from build123d import *

# Parameters (mm, degrees)
CYLINDER002_R     = 0.3
CYLINDER002_DEPTH = 3
CYLINDER001_R     = 0.3
CYLINDER001_DEPTH = 3
BOX001_W          = 1
BOX001_H          = 1
BOX001_DEPTH      = 4
BOX_W             = 1
BOX_H             = 1
BOX_DEPTH         = 4
TORUS_R           = 2.2
CYLINDER_R        = 5.25
CYLINDER_DEPTH    = 14
FILLET_R          = 0.5


with BuildPart() as pin2:
    # Cylinder002 → Cylinder002 (new body)
    with BuildSketch(Plane(origin=(2.5, 0, -3), x_dir=(1, 0, 0), z_dir=(0, 0, 1))):
        Circle(CYLINDER002_R)
    extrude(amount=CYLINDER002_DEPTH)


with BuildPart() as pin1:
    # Cylinder001 → Cylinder001 (new body)
    with BuildSketch(Plane(origin=(-2.5, 0, -3), x_dir=(1, 0, 0), z_dir=(0, 0, 1))):
        Circle(CYLINDER001_R)
    extrude(amount=CYLINDER001_DEPTH)


with BuildPart() as box001:
    # Box001 → Box001 (new body)
    with BuildSketch(Plane(origin=(5, -0.5, 15), x_dir=(1, 0, 0), z_dir=(0, 0, 1))):
        with Locations((0.5, 0.5)):
            Rectangle(BOX001_W, BOX001_H)
    extrude(amount=BOX001_DEPTH)


with BuildPart() as box:
    # Box → Box (new body)
    with BuildSketch(Plane(origin=(5, -0.5, 7), x_dir=(1, 0, 0), z_dir=(0, 0, 1))):
        with Locations((0.5, 0.5)):
            Rectangle(BOX_W, BOX_H)
    extrude(amount=BOX_DEPTH)


with BuildPart() as ring:
    # Torus → Torus (revolve)
    with BuildSketch(Plane(origin=(0, 0, 3.5), x_dir=(1, 0, 0), z_dir=(0, -1, 0))):
        with Locations((7.15, 0)):
            Circle(TORUS_R)
    revolve(axis=Axis((0, 0, 3.5), (0, 0, 1)))


with BuildPart() as obj1:
    # Cylinder → Cylinder (new body)
    with BuildSketch(Plane.XY):
        Circle(CYLINDER_R)
    extrude(amount=CYLINDER_DEPTH)

    # Fillet
    fillet_edges = [obj1.edges().sort_by_distance(p)[0] for p in [
        (-5.25, 0, 14),
        (-5.25, 0, 0),
    ]]
    fillet(fillet_edges, radius=FILLET_R)

    # Cut: cut Ring
    add(ring.part, mode=Mode.SUBTRACT)

    # Cut001: cut Box
    add(box.part, mode=Mode.SUBTRACT)

    # Cut002: cut Box001
    add(box001.part, mode=Mode.SUBTRACT)

    # Fusion: union Pin1+
    add(pin1.part)

    # Fusion001: union Pin2-
    add(pin2.part)


solid = obj1.part
Read the model definition and answer for the solid it produces. Units are mm, in the model's axes. Give positions to 0.01 mm unless a question says otherwise; leave off trailing zeros. Write each loop counter-clockwise with the first axis right and the second up, starting at its lowest first coordinate (ties: lowest second). Pieces come first, ordered by that corner, then holes. Notation, with made-up numbers: (69, 69) - (114, 69) arc R21 cw to (114, 88) - close; hole circle Ø6 at (87, -3). An arc over 180 degrees is marked (long way). Answer in a Markdown table with one row per item. Add a question column.
Item 1: Section C-C, the plane z = 6.75 is taken. Write down the section's boundary in (x, y), and give its area (3 significant figures).
Item 2: Section A-A, the plane y = 0 is taken. Write down the section's boundary in (x, z), and give its area (3 significant figures).
Item 3: Section B-B, the plane x = 0 is taken. Write down the section's boundary in (y, z), and give its area (3 significant figures).
Item 4: Find the intervals of material crossed by L1, parallel to Z at x = 4, y = -2; L2, parallel to Y at x = 2.5, z = -1.5; L3, parallel to X at y = -0.75, z = 2.75, in increasing order.
Item 5: Flat-ended cylindrical pins translate along their axes: P1, Ø3, axis at y = 0, z = 0, coming from the +X side; P2, Ø2, axis at y = 2.5, z = 9.5, coming from the -X side. Find the tip coordinate at first contact, or state that the pin passes through.
Item 6: Determine the mould class of faces 1 (the face through (5, 0, 9)), 2 (the face through (5, 1.6, 9)), 3 (the face through (0, 0, 0)) for opening direction Y: pulls with the +Y half, pulls with the -Y half, needs draft (parallel to the pull), parting line crosses it, or undercut.
Item 7: Section D-D, the plane z = 3.5 is taken. Write down the section's boundary in (x, y).
Recorded:
| question | item | result |
|---|---|---|
| 1 | outline | circle Ø10.5 at (0, 0) |
| 1 | area | 86.6 mm2 |
| 2 | outline | (-5.25, 0.5) arc R0.5 ccw to (-4.75, 0) - (-2.8, 0) - (-2.8, -3) - (-2.2, -3) - (-2.2, 0) - (2.2, 0) - (2.2, -3) - (2.8, -3) - (2.8, 0) - (4.75, 0) arc R0.5 ccw to (5.25, 0.5) - (5.25, 2.39) arc R2.2 cw to (5.25, 4.61) - (5.25, 7) - (5, 7) - (5, 11) - (5.25, 11) - (5.25, 13.5) arc R0.5 ccw to (4.75, 14) - (-4.75, 14) arc R0.5 ccw to (-5.25, 13.5) - (-5.25, 4.61) arc R2.2 cw to (-5.25, 2.39) - close |
| 2 | area | 148 mm2 |
| 3 | outline | (-5.25, 0.5) arc R0.5 ccw to (-4.75, 0) - (4.75, 0) arc R0.5 ccw to (5.25, 0.5) - (5.25, 2.39) arc R2.2 cw to (5.25, 4.61) - (5.25, 13.5) arc R0.5 ccw to (4.75, 14) - (-4.75, 14) arc R0.5 ccw to (-5.25, 13.5) - (-5.25, 4.61) arc R2.2 cw to (-5.25, 2.39) - close |
| 3 | area | 146 mm2 |
| 4 | L1 | z = 0 to 14 |
| 4 | L2 | y = -0.3 to 0.3 |
| 4 | L3 | x = -5.03 to 5.03 |
| 5 | P1 | stops at x = 5.25 |
| 5 | P2 | stops at x = -5.03 |
| 6 | face 1 | undercut |
| 6 | face 2 | parting line crosses it |
| 6 | face 3 | needs draft |
| 7 | outline | circle Ø9.9 at (0, 0) |
